```python
from build123d import *

# Parameters (mm, degrees)
CROQUIS1_R              = 20
CROQUIS1_R_2            = 6.25
CROQUIS1_R_3            = 1.75
SALIENTE_EXTRUIR1_DEPTH = 5
SALIENTE_EXTRUIR2_DEPTH = 5
CROQUIS3_R              = 3.25
CORTAR_EXTRUIR1_DEPTH   = 3
CROQUIS4_R              = 2.5
CORTAR_EXTRUIR2_DEPTH   = 10


with BuildPart() as part:
    # Croquis1 → Saliente-Extruir1 (new, symmetric)
    with BuildSketch(Plane(origin=(0, 0, 0), x_dir=(0, 0, -1), z_dir=(1, 0, 0))):
        Circle(CROQUIS1_R)
        Circle(CROQUIS1_R_2, mode=Mode.SUBTRACT)
        with Locations((0, 13.75)):
            Circle(CROQUIS1_R_3, mode=Mode.SUBTRACT)
        with Locations((11.907849302, 6.875)):
            Circle(CROQUIS1_R_3, mode=Mode.SUBTRACT)
        with Locations((11.907849302, -6.875)):
            Circle(CROQUIS1_R_3, mode=Mode.SUBTRACT)
        with Locations((0, -13.75)):
            Circle(CROQUIS1_R_3, mode=Mode.SUBTRACT)
        with Locations((-11.907849302, -6.875)):
            Circle(CROQUIS1_R_3, mode=Mode.SUBTRACT)
        with Locations((-11.907849302, 6.875)):
            Circle(CROQUIS1_R_3, mode=Mode.SUBTRACT)
    extrude(amount=SALIENTE_EXTRUIR1_DEPTH, both=True)

    # Croquis2 → Saliente-Extruir2 (add, symmetric)
    with BuildSketch(Plane(origin=(0, 0, 0), x_dir=(0, 0, -1), z_dir=(1, 0, 0))):
        with BuildLine():
            Line((-15, -35), (-25, -35))
            Line((-25, -35), (-25, -17.928932188))
            Line((-25, -17.928932188), (-17.228597844, -10.157530032))
            ThreePointArc((-17.228597844, -10.157530032), (-14.142135624, -14.142135624), (-10.157530032, -17.228597844))
            Line((-10.157530032, -17.228597844), (-15, -22.071067812))
            Line((-15, -22.071067812), (-15, -35))
        make_face()
        with BuildLine():
            Line((15, -35), (15, -22.071067812))
            Line((15, -22.071067812), (10.157530032, -17.228597844))
            ThreePointArc((10.157530032, -17.228597844), (14.142135624, -14.142135624), (17.228597844, -10.157530032))
            Line((17.228597844, -10.157530032), (25, -17.928932188))
            Line((25, -17.928932188), (25, -35))
            Line((25, -35), (15, -35))
        make_face()
    extrude(amount=SALIENTE_EXTRUIR2_DEPTH, both=True)

    # Croquis3 → Cortar-Extruir1 (cut)
    with BuildSketch(Plane(origin=(5, 0, 0), x_dir=(0, 0, -1), z_dir=(1, 0, 0))):
        with Locations((0, 13.75)):
            Circle(CROQUIS3_R)
        with Locations((11.907849302, 6.875)):
            Circle(CROQUIS3_R)
        with Locations((11.907849302, -6.875)):
            Circle(CROQUIS3_R)
        with Locations((0, -13.75)):
            Circle(CROQUIS3_R)
        with Locations((-11.907849302, -6.875)):
            Circle(CROQUIS3_R)
        with Locations((-11.907849302, 6.875)):
            Circle(CROQUIS3_R)
    extrude(amount=-CORTAR_EXTRUIR1_DEPTH, mode=Mode.SUBTRACT)

    # Croquis4 → Cortar-Extruir2 (cut)
    with BuildSketch(Plane.XZ.offset(35)):
        with Locations(Location((0, 20, 0), (0, 0, 270))):
            Circle(CROQUIS4_R)
        with Locations(Location((0, -20, 0), (0, 0, 270))):
            Circle(CROQUIS4_R)
    extrude(amount=-CORTAR_EXTRUIR2_DEPTH, mode=Mode.SUBTRACT)


solid = part.part
```
Design review of the part built by this model. Coordinates are the model's own, in mm. A direction names the side the tool comes from. Coordinates: 2 decimals unless noted, no trailing zeros. Order: outer loops, then holes, each group sorted by start corner. A loop starts at its lowest first (then second) coordinate and runs counter-clockwise, first axis right, second up. Notation, with made-up numbers: (15, 46) -> (36, 46) arc R25 ccw to (36, 85) -> close; hole circle Ø10 at (67.5, 67.25). An arc over 180 degrees is marked (long way). One line per item, written item: value. Start each with the question number.
Q1. Insertion check: pin 1 Ø4 at (y, z) = (6.88, -11.91) entering from +X; pin 2 Ø2 at (x, y) = (-1, 1) entering from +Z; pin 3 Ø2 at (x, y) = (-3, -3.5) entering from -Z. Each pin has a flat end and moves straight along its axis. Give the tip position at first contact, or say it passes through.
Q2. Tool access review of faces 4 (the cylindrical face through (0.1, -30.1, -17.5)), 5 (the flat face through (0, -29, -15)), 6 (the flat face through (0.07, -13.99, -21.06)), 7 (the flat face through (-0.07, -14.1, 21.17)), 8 (the cylindrical face through (4, 17, 0)): name each direction out of +Z, -Z, +X, -X, +Y, -Y from which nothing blocks a thin tool from reaching the whole face with its end or side.
Q3. Take a section at B-B, the plane y = -26.5. State the section outline as (x, z) points, then the cut area to 3 significant figures.
Q4. Take a section at A-A, the plane y = 0. State the section outline as (x, z) points, then the cut area to 3 significant figures.
Q5. Take a section at C-C, the plane z = 0. State the section outline as (x, y) points, then the cut area to 3 significant figures.
Q6. Take a section at D-D, the plane x = 0. State the section outline as (y, z) points (3 decimals), then the cut area to 3 significant figures.
Q7. Mouldability with a two-part tool opening along X and no side actions: class faces 1 (the flat face through (2, 12, -1)), 2 (the cylindrical face through (3.521, -10.528, 0.423)), 3 (the flat face through (0, -25, 20)) as pulls with the +X half, pulls with the -X half, needs draft (parallel to the pull), parting line crosses it, or undercut.
Q8. For probe 1 along Y at (x, z) = (-3.5, 13.5); probe 2 along Z at (x, y) = (4.25, -9); probe 3 along Z at (x, y) = (-1.75, -8), list the stretches that pass through material, from the lowest coordinate up.
Values follow:
1. pin 1: stops at x = 2
1. pin 2: stops at z = 20
1. pin 3: stops at z = -19.84
2. face 4: -Y
2. face 5: +X, -X, -Y
2. face 6: -Z, +X, -X
2. face 7: +Z, +X, -X
2. face 8: +X
3. outline: (-5, -25) -> (5, -25) -> (5, -15) -> (-5, -15) -> close; (-5, 15) -> (5, 15) -> (5, 25) -> (-5, 25) -> close; hole circle Ø5 at (0, -20); hole circle Ø5 at (0, 20)
3. area: 161 mm2
4. outline: (-5, -20) -> (5, -20) -> (5, -6.25) -> (-5, -6.25) -> close; (-5, 6.25) -> (5, 6.25) -> (5, 20) -> (-5, 20) -> close
4. area: 275 mm2
5. outline: (-5, -20) -> (5, -20) -> (5, -17) -> (2, -17) -> (2, -15.5) -> (-5, -15.5) -> close; (-5, -12) -> (2, -12) -> (2, -10.5) -> (5, -10.5) -> (5, -6.25) -> (-5, -6.25) -> close; (-5, 6.25) -> (5, 6.25) -> (5, 10.5) -> (2, 10.5) -> (2, 12) -> (-5, 12) -> close; (-5, 15.5) -> (2, 15.5) -> (2, 17) -> (5, 17) -> (5, 20) -> (-5, 20) -> close
5. area: 187 mm2
6. outline: (-35, -25) -> (-17.929, -25) -> (-10.158, -17.229) arc R20 ccw (long way) to (-10.158, 17.229) -> (-17.929, 25) -> (-35, 25) -> (-35, 22.5) -> (-25, 22.5) -> (-25, 17.5) -> (-35, 17.5) -> (-35, 15) -> (-22.071, 15) -> (-17.229, 10.158) arc R20 ccw to (-17.229, -10.158) -> (-22.071, -15) -> (-35, -15) -> (-35, -17.5) -> (-25, -17.5) -> (-25, -22.5) -> (-35, -22.5) -> close; hole circle Ø3.5 at (-13.75, 0); hole circle Ø3.5 at (-6.875, -11.908); hole circle Ø3.5 at (-6.875, 11.908); hole circle Ø12.5 at (0, 0); hole circle Ø3.5 at (6.875, -11.908); hole circle Ø3.5 at (6.875, 11.908); hole circle Ø3.5 at (13.75, 0)
6. area: 1,450 mm2
7. face 1: pulls with the +X half
7. face 2: needs draft
7. face 3: undercut
8. probe 1: y = -20.57 to -7.6, -6.15 to 6.15, 7.6 to 14.76
8. probe 2: z = -17.86 to -14.37, -9.45 to 9.45, 14.37 to 17.86
8. probe 3: z = -18.33 to -13.25, -10.57 to 10.57, 13.25 to 18.33
